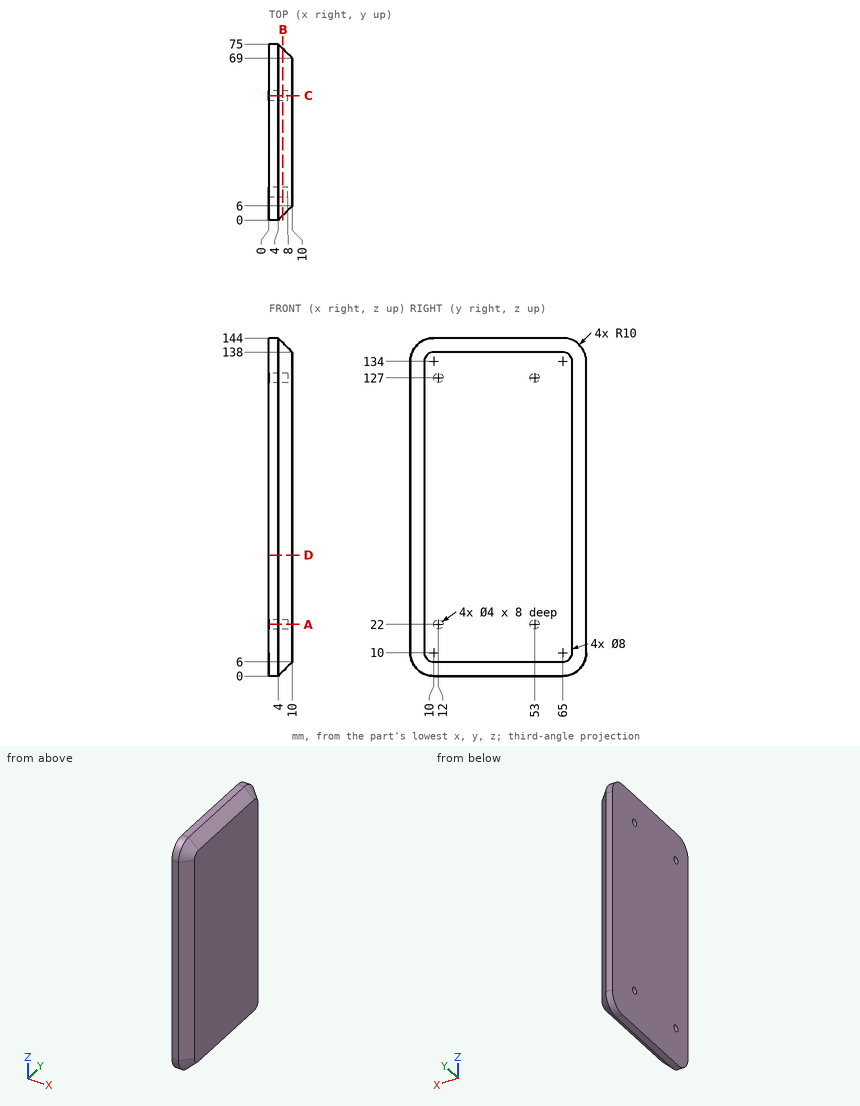
Design review of the part shown in the three views and the two pictorial views. Dimensions are in mm from the part's minimum x, y and z. Coordinates: 2 decimals unless noted, no trailing zeros. Write each loop counter-clockwise with the first axis right and the second up, starting at its lowest first coordinate (ties: lowest second). Pieces come first, ordered by that corner, then holes.
1) We need section C-C on y = 53. State the section outline as (x, z) points, then the cut area to 3 significant figures.
2) We need section B-B on x = 6. State the section outline as (y, z) points, then the cut area to 3 significant figures.
3) Clearance check with flat-ended pins moving along their axes: pin 1 Ø4 at (x, y) = (7.5, 26.5) entering from +Z; pin 2 Ø1 at (x, z) = (7.5, 16.5) entering from +Y; pin 3 Ø2.5 at (y, z) = (53, 22) entering from -X. State where each tip first meets the part, or that it passes through.
4) To check wall thickness, follow probe 1 along Z at (x, y) = (2.5, 53); probe 2 along Z at (x, y) = (5, 12); probe 3 along Y at (x, z) = (3.5, 126). State the ranges of each line that lie inside material, in increasing order.
5) We need section A-A on z = 22. State the section outline as (x, y) points, then the cut area to 3 significant figures.
6) We need section D-D on z = 51.5. State the section outline as (x, y) points.
Answer list:
1. outline: (0, 0) - (4, 0) - (10, 6) - (10, 138) - (4, 144) - (0, 144) - (0, 129) - (8, 129) - (8, 125) - (0, 125) - (0, 24) - (8, 24) - (8, 20) - (0, 20) - close
1. area: 1,340 mm2
2. outline: (2, 10) arc R8 ccw to (10, 2) - (65, 2) arc R8 ccw to (73, 10) - (73, 134) arc R8 ccw to (65, 142) - (10, 142) arc R8 ccw to (2, 134) - close; hole circle Ø4 at (12, 22); hole circle Ø4 at (12, 127); hole circle Ø4 at (53, 22); hole circle Ø4 at (53, 127)
2. area: 9,830 mm2
3. pin 1: stops at z = 142.5
3. pin 2: stops at y = 72
3. pin 3: stops at x = 8
4. probe 1: z = 0 to 20, 24 to 125, 129 to 144
4. probe 2: z = 1 to 20, 24 to 125, 129 to 143
4. probe 3: y = 0 to 10.27, 13.73 to 51.27, 54.73 to 75
5. outline: (0, 0) - (4, 0) - (10, 6) - (10, 69) - (4, 75) - (0, 75) - (0, 55) - (8, 55) - (8, 51) - (0, 51) - (0, 14) - (8, 14) - (8, 10) - (0, 10) - close
5. area: 650 mm2
6. outline: (0, 0) - (4, 0) - (10, 6) - (10, 69) - (4, 75) - (0, 75) - close
